Here's how the part is built. I have some questions about the finished solid (model axes, mm). Face numbers are marked on the shaded views. A direction names the side the tool comes from. Round coordinates to 2 decimals unless told otherwise and drop trailing zeros. Loops run counter-clockwise (first coordinate to the right, second up) from the corner with the lowest first, then second, coordinate; pieces in that order, holes last. Notation, with made-up numbers: (81.5, -14) - (95.5, -14) arc R21 ccw to (95.5, 17) - close; hole circle Ø4 at (-24.75, -12). An arc over 180 degrees is marked (long way). Answer as a JSON object with one key per item and string values. Group by question number.
1) If we mould it in two halves opening along X, with no side actions, what happens to the marked faces 3, 4 and 5? For each: pulls with the +X half, pulls with the -X half, needs draft (parallel to the pull), parting line crosses it, or undercut.
2) I want a section at A-A, the plane z = -29. Please give me the cut outline in (x, y), then the cut area to 3 significant figures.
3) Which directions (+Z, -Z, +X, -X, +Y, -Y) give clear straight access to the entire face, cutting with the end or side of a thin tool? Please do the marked faces 1 and 2.
4) I want a section at B-B, the plane y = 18.25. Please give me the cut outline in (x, z), then the cut area to 3 significant figures.
5) If I drill on line 1 along X through (y, z) = (17, 9.5); line 2 along Y through (x, z) = (56.3, 29); line 3 along Z through (x, y) = (24.5, 13.5), over which ranges is the centre line in solid material (lowest first)? Write a range as [from, to].
6) I want a section at C-C, the plane x = 10. Please give me the cut outline in (y, z).
7) I want a section at D-D, the plane y = 8. Please give me the cut outline in (x, z), then the cut area to 3 significant figures.
8) Will these pins go through, and if not, where does the flat tip stop? P1, Ø1.5, axis at x = 27.5, z = -16, coming from the +Y side; P2, Ø5, axis at y = 8, z = 29, coming from the -X side.
from build123d import *

# Parameters (mm, degrees)
SKETCH1_W                = 108
SKETCH1_H                = 68
BOSS_EXTRUDE1_DEPTH      = 3
SKETCH2_W                = 114
SKETCH2_H                = 74
SKETCH2_W_2              = 108
SKETCH2_H_2              = 68
BOSS_EXTRUDE2_DEPTH      = 25
BOSS_EXTRUDE2_DEPTH_BACK = 3
SKETCH4_W                = 114
SKETCH4_H                = 74
SKETCH4_W_2              = 111
SKETCH4_H_2              = 71
BOSS_EXTRUDE3_DEPTH      = 2
SKETCH5_R                = 2
CUT_EXTRUDE1_DEPTH       = 4
SKETCH6_W                = 13
SKETCH6_H                = 3
CUT_EXTRUDE2_DEPTH       = 31
MIRROR2_COPY_1_SKETCH_R  = 2
MIRROR2_COPY_1_DEPTH     = 4
SKETCH7_W                = 13
SKETCH7_H                = 3
CUT_EXTRUDE3_DEPTH       = 10
CUT_EXTRUDE4_DEPTH       = 2


with BuildPart() as part:
    # Sketch1 → Boss-Extrude1 (new body)
    with BuildSketch(Plane(origin=(0, 0, 0), x_dir=(1, 0, 0), z_dir=(0, 1, 0))):
        Rectangle(SKETCH1_W, SKETCH1_H)
    extrude(amount=BOSS_EXTRUDE1_DEPTH)

    # Sketch2 → Boss-Extrude2 (add, two sides)
    with BuildSketch(Plane(origin=(0, 3, 0), x_dir=(1, 0, 0), z_dir=(0, 1, 0))) as boss_extrude2_sk:
        Rectangle(SKETCH2_W, SKETCH2_H)
        Rectangle(SKETCH2_W_2, SKETCH2_H_2, mode=Mode.SUBTRACT)
    extrude(amount=BOSS_EXTRUDE2_DEPTH)
    extrude(boss_extrude2_sk.sketch, amount=-BOSS_EXTRUDE2_DEPTH_BACK)

    # Sketch4 → Boss-Extrude3 (add)
    with BuildSketch(Plane(origin=(0, 28, 0), x_dir=(1, 0, 0), z_dir=(0, 1, 0))):
        Rectangle(SKETCH4_W, SKETCH4_H)
        Rectangle(SKETCH4_W_2, SKETCH4_H_2, mode=Mode.SUBTRACT)
    extrude(amount=BOSS_EXTRUDE3_DEPTH)

    # Sketch5 → Cut-Extrude1 (cut, through all)
    with BuildSketch(Plane(origin=(-54, 0, 0), x_dir=(0, 0, -1), z_dir=(1, 0, 0))):
        with Locations((29, 8)):
            Circle(SKETCH5_R)
    cut_extrude1 = extrude(amount=-CUT_EXTRUDE1_DEPTH, mode=Mode.SUBTRACT)

    # Sketch6 → Cut-Extrude2 (cut, through all)
    with BuildSketch(Plane.XZ):
        with Locations((20.5, 22.5)):
            Rectangle(SKETCH6_W, SKETCH6_H)
        with Locations((37.5, 22.5)):
            Rectangle(SKETCH6_W, SKETCH6_H)
        with Locations((20.5, 15.5)):
            Rectangle(SKETCH6_W, SKETCH6_H)
        with Locations((37.5, 15.5)):
            Rectangle(SKETCH6_W, SKETCH6_H)
        with Locations((20.5, 8.5)):
            Rectangle(SKETCH6_W, SKETCH6_H)
        with Locations((37.5, 8.5)):
            Rectangle(SKETCH6_W, SKETCH6_H)
        with Locations((20.5, 1.5)):
            Rectangle(SKETCH6_W, SKETCH6_H)
        with Locations((37.5, 1.5)):
            Rectangle(SKETCH6_W, SKETCH6_H)
        with Locations((20.5, -5.5)):
            Rectangle(SKETCH6_W, SKETCH6_H)
        with Locations((37.5, -5.5)):
            Rectangle(SKETCH6_W, SKETCH6_H)
        with Locations((20.5, -12.5)):
            Rectangle(SKETCH6_W, SKETCH6_H)
        with Locations((37.5, -12.5)):
            Rectangle(SKETCH6_W, SKETCH6_H)
        with Locations((20.5, -19.5)):
            Rectangle(SKETCH6_W, SKETCH6_H)
        with Locations((37.5, -19.5)):
            Rectangle(SKETCH6_W, SKETCH6_H)
    extrude(amount=-CUT_EXTRUDE2_DEPTH, mode=Mode.SUBTRACT)

    # Mirror1: Cut-Extrude1 across plane
    add(cut_extrude1.mirror(Plane.XY), mode=Mode.SUBTRACT)

    # Mirror2: Cut-Extrude1 across plane
    add(cut_extrude1.mirror(Plane(origin=(0, 0, 0), x_dir=(0, 0, 1), z_dir=(1, 0, 0))), mode=Mode.SUBTRACT)

    # Mirror2 copy 1 sketch → Mirror2 copy 1 (cut, through all)
    with BuildSketch(Plane.ZY.offset(-54)):
        with Locations((29, 8)):
            Circle(MIRROR2_COPY_1_SKETCH_R)
    extrude(amount=-MIRROR2_COPY_1_DEPTH, mode=Mode.SUBTRACT)

    # Sketch7 → Cut-Extrude3 (cut)
    with BuildSketch(Plane(origin=(0, 3, 0), x_dir=(1, 0, 0), z_dir=(0, 1, 0))):
        with Locations((-24, 17.5)):
            Rectangle(SKETCH7_W, SKETCH7_H)
        with Locations((-24, 4.583391615)):
            Rectangle(SKETCH7_W, SKETCH7_H)
        with Locations((-24, -8.333216771)):
            Rectangle(SKETCH7_W, SKETCH7_H)
        with Locations((-24, -21.249825156)):
            Rectangle(SKETCH7_W, SKETCH7_H)
    extrude(amount=-CUT_EXTRUDE3_DEPTH, mode=Mode.SUBTRACT)

    # Sketch8 → Cut-Extrude4 (cut)
    with BuildSketch(Plane(origin=(0, 28, 0), x_dir=(1, 0, 0), z_dir=(0, 1, 0))):
        Polygon((-54, 34), (-50.5, 34), (-50.5, 35.5), (-55.5, 35.5), (-55.5, 30.5), (-54, 30.5), align=None)
        Polygon((54, -34), (54, -30.5), (55.5, -30.5), (55.5, -35.5), (50.5, -35.5), (50.5, -34), align=None)
    extrude(amount=-CUT_EXTRUDE4_DEPTH, mode=Mode.SUBTRACT)


solid = part.part
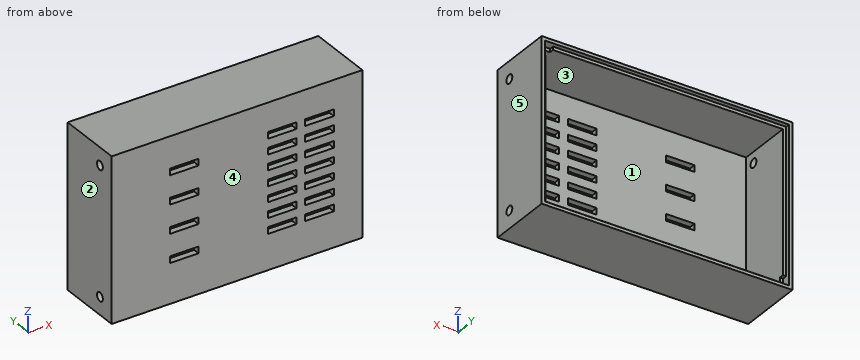
Outcome:
{
 "1": {"face 3": "undercut", "face 4": "needs draft", "face 5": "pulls with the +X half"},
 "2": {"outline": "(-57, 0) - (57, 0) - (57, 6) - (54, 6) - (54, 3) - (-54, 3) - (-54, 6) - (-57, 6) - close; (-57, 10) - (-54, 10) - (-54, 28) - (-55.5, 28) - (-55.5, 30) - (-57, 30) - close; (54, 10) - (57, 10) - (57, 30) - (55.5, 30) - (55.5, 28) - (54, 28) - close", "area": "474 mm^2"},
 "3": {"face 1": "+Y", "face 2": "+Z, -Z, -X, +Y, -Y"},
 "4": {"outline": "(-57, -37) - (57, -37) - (57, 37) - (-57, 37) - close; hole (-54, -34) - (54, -34) - (54, 34) - (-54, 34) - close", "area": "1,090 mm^2"},
 "5": {"line 1": "[-57, -54], [54, 57]", "line 2": "[0, 6], [10, 30]", "line 3": "[-37, -34], [34, 37]"},
 "6": {"outline": "(0, -37) - (30, -37) - (30, -35.5) - (28, -35.5) - (28, -34) - (3, -34) - (3, 34) - (28, 34) - (28, 35.5) - (30, 35.5) - (30, 37) - (0, 37) - close"},
 "7": {"outline": "(-57, -37) - (57, -37) - (57, -31) - (54, -31) - (54, -34) - (-54, -34) - (-54, -31) - (-57, -31) - close; (-57, -27) - (-54, -27) - (-54, 27) - (-57, 27) - close; (-57, 31) - (-54, 31) - (-54, 34) - (54, 34) - (54, 31) - (57, 31) - (57, 37) - (-57, 37) - close; (54, -27) - (57, -27) - (57, 27) - (54, 27) - close", "area": "1,040 mm^2"},
 "8": {"P1": "y = 3", "P2": "x = -57"}
}
